Could you check a few things on this model? Use its own coordinates, in mm. Face numbers are marked on the shaded views. A direction names the side the tool comes from. Round coordinates to 2 decimals unless told otherwise and drop trailing zeros. Write each loop counter-clockwise with the first axis right and the second up, starting at its lowest first coordinate (ties: lowest second). Pieces come first, ordered by that corner, then holes. Notation, with made-up numbers: (19, -10.5) -> (70, -10.5) arc R15 ccw to (70, 5.5) -> close; hole circle Ø9 at (17, 36.5). An arc over 180 degrees is marked (long way). Answer in a Markdown table with one row per item.
Autodesk Inventor part; units mm, degrees
ref_plane "YZ Plane" through (0, 0, 0) normal (1, 0, 0) x (0, 1, 0)
ref_plane "XZ Plane" through (0, 0, 0) normal (0, 1, 0) x (-1, 0, 0)
ref_plane "XY Plane" through (0, 0, 0) normal (0, 0, 1) x (1, 0, 0)
sketch "Sketch1" plane through (0, 0, 0) normal (0, 1, 0) x (-1, 0, 0)
  circle A0 centre (0, 0) radius 38.5
  circle A1 centre (0, 0) radius 41
  dimension "d0" = 77
  dimension "d1" = 82
extrude "Extrusion3" add sketch "Sketch1" along normal blind 3 contours A0
sketch "Sketch3" plane through (0, 0, 0) normal (0, 1, 0) x (-1, 0, 0)
  circle A0 centre (0, 0) radius 41
  circle A1 centre (0, 0) radius 38.5
  dimension "d9" = 82
  dimension "d10" = 77
extrude "Extrusion4" add sketch "Sketch3" along normal blind 15
sketch "Sketch4" plane through (0, 3, 0) normal (0, 1, 0) x (1, 0, 0)
  line L0 (0, 0) -> (41, 0)
  circle A0 centre (0, 0) radius 41
  line L1 (0, 0) -> (28.9914, 28.9914)
  line L2 (0, 0) -> (41, 0) construction
  arc A1 (41, 0) -> (28.9914, 28.9914) centre (0, 0) ccw
  dimension "d13" = 41
  dimension "d14" = 45
extrude "Extrusion5" cut sketch "Sketch4" along normal blind 15 contours L1 A0 L0 picked at (21.0272, 17.2566)
properties part number "mainbody"
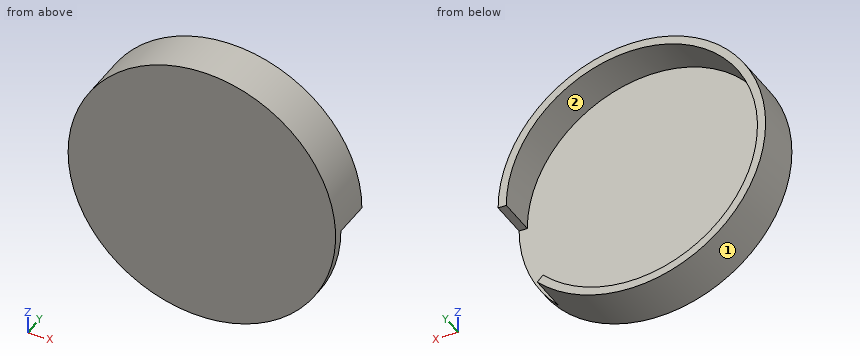
1) Imagine slicing it at B-B, the plane z = 5. Please give me the cut outline in (x, y).
Findings:
| item | result |
|---|---|
| outline | (-40.69, 0) -> (40.69, 0) -> (40.69, 15) -> (38.17, 15) -> (38.17, 3) -> (-38.17, 3) -> (-38.17, 15) -> (-40.69, 15) -> close |
2) For the marked faces 1 and 2, which set-ups out of +Z, -Z, +X, -X, +Y, -Y let a thin tool reach every point of the face, with its end or its side?
Findings:
| item | result |
|---|---|
| face 1 | +Y, -Y |
| face 2 | +Y |
3) Imagine slicing it at C-C, the plane y = 5.25. Please give me the cut outline in (x, z).
Findings:
| item | result |
|---|---|
| outline | (27.22, -27.22) arc R38.5 cw (long way) to (38.5, 0) -> (41, 0) arc R41 ccw (long way) to (28.99, -28.99) -> close |
4) Imagine slicing it at D-D, the plane z = -21.5. Please give me the cut outline in (x, y).
Findings:
| item | result |
|---|---|
| outline | (-34.91, 0) -> (34.91, 0) -> (34.91, 3) -> (-31.94, 3) -> (-31.94, 15) -> (-34.91, 15) -> close |
5) Imagine slicing it at A-A, the plane x = 0. Please give me the cut outline in (y, z).
Findings:
| item | result |
|---|---|
| outline | (0, -41) -> (15, -41) -> (15, -38.5) -> (3, -38.5) -> (3, 38.5) -> (15, 38.5) -> (15, 41) -> (0, 41) -> close |
6) Please list where these lines run through material, in increasing order: line 1 (Z direction, x = 0, y = 5.5); line 2 (Z direction, x = -18, y = 11.75); line 3 (Y direction, x = 12.5, z = 22).
Findings:
| item | result |
|---|---|
| line 1 | z = -41 to -38.5, 38.5 to 41 |
| line 2 | z = -36.84 to -34.03, 34.03 to 36.84 |
| line 3 | y = 0 to 3 |
7) For pin 1 (2 mm diameter, centred on x = 23.5, y = 8.5, fed in from -Z); pin 2 (1.5 mm diameter, centred on y = 5, z = 15, fed in from +X); pin 3 (1 mm diameter, centred on x = 19.5, z = 3, fed in from -Y); pin 4 (2 mm diameter, centred on x = 27, z = 15, fed in from +Y), each with a flat end and sliding along its axis, tell me the tip position at first contact or that it passes through.
Findings:
| item | result |
|---|---|
| pin 1 | stops at z = -34.27 |
| pin 2 | stops at x = 38.44 |
| pin 3 | stops at y = 0 |
| pin 4 | stops at y = 3 |
